```python
from build123d import *

# Parameters (mm, degrees)
SKETCH_R                    = 175
SKETCH_R_2                  = 7.5
PAD_DEPTH                   = 20.5
SKETCH009_R                 = 3
POCKET_DEPTH                = 5
SKETCH009_POLARPATTERN_2_R  = 3
POCKET_POLARPATTERN_2_DEPTH = 5
POLARPATTERN001_COUNT       = 8
POCKET001_DEPTH             = 20.501
FILLET001_R                 = 1


with BuildPart() as part:
    # Sketch → Pad (new body)
    with BuildSketch(Plane.XY):
        Circle(SKETCH_R)
        Circle(SKETCH_R_2, mode=Mode.SUBTRACT)
    extrude(amount=PAD_DEPTH)

    # Sketch009 → Pocket (cut)
    with BuildSketch(Plane.XY):
        with Locations((25.420601, 160.499355)):
            Circle(SKETCH009_R)
    pocket = extrude(amount=POCKET_DEPTH, mode=Mode.SUBTRACT)

    # Sketch009 PolarPattern 2 → Pocket PolarPattern 2 (cut)
    with BuildSketch(Plane(origin=(0, 0, 0), x_dir=(0.987688, -0.156434, 0), z_dir=(0, 0, 1))):
        with Locations((25.420601, 160.499355)):
            Circle(SKETCH009_POLARPATTERN_2_R)
    pocket_polarpattern_2 = extrude(amount=POCKET_POLARPATTERN_2_DEPTH, mode=Mode.SUBTRACT)

    # PolarPattern001: Pocket, Pocket PolarPattern 2 ×8 about axis
    polarpattern001_axis = Axis((0, 0, 0), (0, 0, 1))
    for i in range(1, POLARPATTERN001_COUNT):
        add(pocket.rotate(polarpattern001_axis, i * 360 / POLARPATTERN001_COUNT), mode=Mode.SUBTRACT)
        add(pocket_polarpattern_2.rotate(polarpattern001_axis, i * 360 / POLARPATTERN001_COUNT), mode=Mode.SUBTRACT)

    # Sketch010 → Pocket001 (cut, through all)
    with BuildSketch(Plane.XY):
        with BuildLine():
            ThreePointArc((-3.1, 0), (0, -3.1), (3.1, 0))
            Line((3.1, 0), (3.1, 8))
            ThreePointArc((3.1, 8), (0, 11.1), (-3.1, 8))
            Line((-3.1, 8), (-3.1, 0))
        make_face()
    extrude(amount=POCKET001_DEPTH, mode=Mode.SUBTRACT)

    # Fillet001
    fillet001_edges = [part.edges().sort_by_distance(p)[0] for p in [
        (-3.1, 6.829348, 10.25),
        (3.1, 6.829348, 10.25),
    ]]
    fillet(fillet001_edges, radius=FILLET001_R)


solid = part.part
```
Verification items for the finished model (mm, model axes). Round coordinates to 2 decimals unless told otherwise and drop trailing zeros. Write each loop counter-clockwise with the first axis right and the second up, starting at its lowest first coordinate (ties: lowest second). Pieces come first, ordered by that corner, then holes.
1. Section check A-A on y = 0. Enter the section's corners in (x, z).
2. Section check B-B on z = 10.5. Enter the section's corners in (x, y).
3. Section check C-C on y = -66. Enter the section's corners in (x, z).
4. Section check D-D on x = 102.5. Enter the section's corners in (y, z), plus the area to 3 significant figures.
5. Draft check along X on faces 1 (the flat face through (36, 2, 0)), 2 (the cylindrical face through (-0.277, -7.495, 10.106)), 3 (the cylindrical face through (-128.982, 118.273, 10.106)). Enter one of: +X half, -X half, draft (parallel to the pull), parting line (faces both ways), or undercut.
6. Scan lines: L1, parallel to Y at x = 146, z = 3; L2, parallel to X at y = 57, z = 4.5; L3, parallel to Y at x = -115, z = 11.25. Record each from-to range of solid material in increasing order.
7. Gauge pin test, flat ends, axial feed: P1, Ø2, axis at x = 135.5, z = 18, coming from the +Y side; P2, Ø1.8, axis at x = 132.5, y = 94, coming from the -Z side; P3, Ø6, axis at x = 132.5, z = 11.5, coming from the +Y side. Record the tip position at first contact, or that the pin passes through.
Answer:
1. outline: (-175, 0) - (-7.5, 0) - (-7.5, 20.5) - (-175, 20.5) - close; (7.5, 0) - (175, 0) - (175, 20.5) - (7.5, 20.5) - close
2. outline: circle Ø350 at (0, 0); hole (-3.62, 6.57) arc R7.5 ccw (long way) to (3.62, 6.57) arc R1 cw to (3.1, 7.45) - (3.1, 8) arc R3.1 ccw to (-3.1, 8) - (-3.1, 7.45) arc R1 cw to start
3. outline: (-162.08, 0) - (162.08, 0) - (162.08, 20.5) - (-162.08, 20.5) - close
4. outline: (-141.84, 0) - (141.84, 0) - (141.84, 20.5) - (-141.84, 20.5) - close
4. area: 5,820 mm2
5. face 1: draft
5. face 2: undercut
5. face 3: parting line
6. L1: y = -96.48 to 71.03, 76.52 to 96.48
6. L2: x = -165.46 to 165.46
6. L3: y = -131.91 to 131.91
7. P1: stops at y = 111.96
7. P2: stops at z = 5
7. P3: stops at y = 117.71
